Source: CAD feature listing. Evaluate the final solid. Frame: model axes, mm. Face numbers are marked on the shaded views. A direction names the side the tool comes from. Coordinates: 2 decimals unless noted, no trailing zeros. Order: outer loops, then holes, each group sorted by start corner. A loop starts at its lowest first (then second) coordinate and runs counter-clockwise, first axis right, second up.
```python
from build123d import *

# Parameters (mm, degrees)
BOSS_EXTRU_1_DEPTH      = 180
ESQUISSE2_R             = 3
ENL_V_MAT_EXTRU_1_DEPTH = 180
ESQUISSE3_R             = 2.5
ENL_V_MAT_EXTRU_2_DEPTH = 180
CONG_1_R                = 2


with BuildPart() as part:
    # Esquisse1 → Boss.-Extru.1 (new body)
    with BuildSketch(Plane.XY):
        Polygon((0, 0), (0, -30), (3, -30), (3, -3), (30, -3), (30, 0), align=None)
    extrude(amount=BOSS_EXTRU_1_DEPTH)

    # Esquisse2 → Enlèv. mat.-Extru.1 (cut)
    with BuildSketch(Plane(origin=(3, 0, 0), x_dir=(0, 0, -1), z_dir=(1, 0, 0))):
        with Locations((-30, -15)):
            Circle(ESQUISSE2_R)
        with Locations((-150, -15)):
            Circle(ESQUISSE2_R)
    extrude(amount=-ENL_V_MAT_EXTRU_1_DEPTH, mode=Mode.SUBTRACT)

    # Esquisse3 → Enlèv. mat.-Extru.2 (cut)
    with BuildSketch(Plane.XZ.offset(3)):
        with Locations((15, 150)):
            Circle(ESQUISSE3_R)
        with Locations((15, 30)):
            Circle(ESQUISSE3_R)
    extrude(amount=-ENL_V_MAT_EXTRU_2_DEPTH, mode=Mode.SUBTRACT)

    # Congé1
    cong_1_edges = [part.edges().sort_by_distance(p)[0] for p in [
        (3, -3, 90),
        (0, 0, 90),
    ]]
    fillet(cong_1_edges, radius=CONG_1_R)


solid = part.part
```
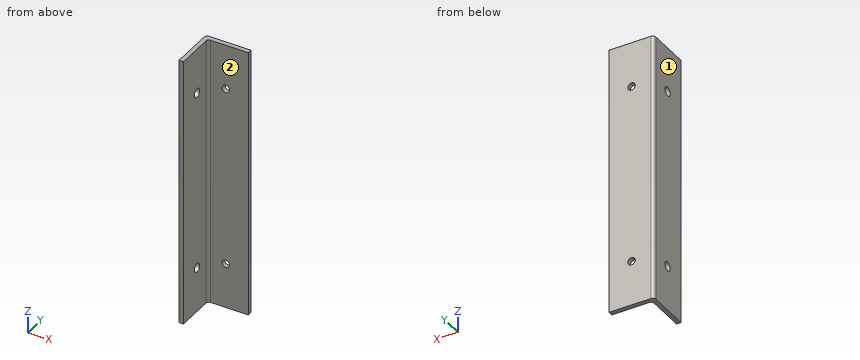
Q1. Pin query (flat end, axial travel): P1, Ø6, axis at x = 13.5, z = 88, coming from the -Y side; P2, Ø8, axis at y = -15, z = 150, coming from the +X side. Return the tip coordinate at first contact, or that it passes through.
Solutions:
P1: stops at y = -3
P2: stops at x = 3
Q2. Material intervals for line 1 along Z through (x, y) = (15, -1.2); line 2 along Y through (x, z) = (2.35, 150); line 3 along X through (y, z) = (-5.5, 63.5), sorted ascending.
Solutions:
line 1: z = 0 to 27.5, 32.5 to 147.5, 152.5 to 180
line 2: y = -30 to -18, -12 to 0
line 3: x = 0 to 3
Q3. Section query A-A on z = 150. Output: boundary loops of the cut face in (x, y), plus the area to 3 significant figures.
Solutions:
outline: (0, -30) - (3, -30) - (3, -18) - (0, -18) - close; (0, -12) - (3, -12) - (3, -5) arc R2 cw to (5, -3) - (12.5, -3) - (12.5, 0) - (2, 0) arc R2 ccw to (0, -2) - close; (17.5, -3) - (30, -3) - (30, 0) - (17.5, 0) - close
area: 138 mm2
Q4. Section query D-D on y = -6.75. Output: boundary loops of the cut face in (x, z).
Solutions:
outline: (0, 0) - (3, 0) - (3, 180) - (0, 180) - close
Q5. Section query C-C on x = 15. Output: boundary loops of the cut face in (y, z).
Solutions:
outline: (-3, 0) - (0, 0) - (0, 27.5) - (-3, 27.5) - close; (-3, 32.5) - (0, 32.5) - (0, 147.5) - (-3, 147.5) - close; (-3, 152.5) - (0, 152.5) - (0, 180) - (-3, 180) - close
Q6. Set-up query: the marked faces 1 and 2. Return all of +Z, -Z, +X, -X, +Y, -Y with unobstructed straight access to the full face (end or side cutting, diameter ignored); none if empty.
Solutions:
face 1: +Z, -Z, -X, +Y, -Y
face 2: +Z, -Z, +X, -Y
Q7. Section query B-B on y = -15. Output: boundary loops of the cut face in (x, z).
Solutions:
outline: (0, 0) - (3, 0) - (3, 27) - (0, 27) - close; (0, 33) - (3, 33) - (3, 147) - (0, 147) - close; (0, 153) - (3, 153) - (3, 180) - (0, 180) - close
